from build123d import *

# Parameters (mm, degrees)
BOSS_EXTRUDE1_DEPTH = 20
FILLET1_R           = 50
FILLET2_R           = 5
SKETCH3_R           = 1.5
CUT_EXTRUDE1_DEPTH  = 20
SKETCH4_R           = 2.5
CUT_EXTRUDE2_DEPTH  = 10
SKETCH5_R           = 1
CUT_EXTRUDE3_DEPTH  = 20


with BuildPart() as part:
    # Sketch2 → Boss-Extrude1 (new body)
    with BuildSketch(Plane(origin=(0, 0, 0), x_dir=(1, 0, 0), z_dir=(0, 1, 0))):
        with BuildLine():
            Line((25, -30), (60, -30))
            Line((60, -30), (60, 0))
            Line((60, 0), (45, 0))
            Line((45, 0), (0, 10))
            Line((0, 10), (-45, 0))
            Line((-45, 0), (-60, 0))
            Line((-60, 0), (-60, -30))
            Line((-60, -30), (-25, -30))
            add(Edge.make_bspline(
                [(0, 0), (-26.0775505, -1.658562804), (-25, -30)],
                knots=[0, 0, 0, 1, 1, 1], degree=2))
            add(Edge.make_bspline(
                [(0, 0), (26.0775505, -1.658562804), (25, -30)],
                knots=[0, 0, 0, 1, 1, 1], degree=2))
        make_face()
    extrude(amount=BOSS_EXTRUDE1_DEPTH)

    # Fillet1
    fillet1_edges = [part.edges().sort_by_distance(p)[0] for p in [
        (0, 10, -10),
    ]]
    fillet(fillet1_edges, radius=FILLET1_R)

    # Fillet2
    fillet2_edges = [part.edges().sort_by_distance(p)[0] for p in [
        (-60, 10, 0),
        (60, 10, 0),
    ]]
    fillet(fillet2_edges, radius=FILLET2_R)

    # Sketch3 → Cut-Extrude1 (cut)
    with BuildSketch(Plane.XY.offset(30)):
        with Locations((50, 10)):
            Circle(SKETCH3_R)
    cut_extrude1 = extrude(amount=-CUT_EXTRUDE1_DEPTH, mode=Mode.SUBTRACT)

    # Sketch4 → Cut-Extrude2 (cut)
    with BuildSketch(Plane(origin=(0, 0, 0), x_dir=(-1, 0, 0), z_dir=(0, 0, -1))):
        with Locations((-50, 10)):
            Circle(SKETCH4_R)
    cut_extrude2 = extrude(amount=-CUT_EXTRUDE2_DEPTH, mode=Mode.SUBTRACT)

    # Mirror1: Cut-Extrude1, Cut-Extrude2 across plane
    add(cut_extrude1.mirror(Plane(origin=(0, 0, 0), x_dir=(0, 0, 1), z_dir=(1, 0, 0))), mode=Mode.SUBTRACT)
    add(cut_extrude2.mirror(Plane(origin=(0, 0, 0), x_dir=(0, 0, 1), z_dir=(1, 0, 0))), mode=Mode.SUBTRACT)

    # Sketch5 → Cut-Extrude3 (cut)
    with BuildSketch(Plane(origin=(0, 20, 0), x_dir=(1, 0, 0), z_dir=(0, 1, 0))):
        with Locations(Location((30, -27, 0), (0, 0, 270))):
            Circle(SKETCH5_R)
    cut_extrude3 = extrude(amount=-CUT_EXTRUDE3_DEPTH, mode=Mode.SUBTRACT)

    # Mirror2: Cut-Extrude3 across plane
    add(cut_extrude3.mirror(Plane(origin=(0, 0, 0), x_dir=(0, 0, 1), z_dir=(1, 0, 0))), mode=Mode.SUBTRACT)


solid = part.part
Build history of the part. All positions in model axes, mm. A direction names the side the tool comes from. Coordinates: 2 decimals unless noted, no trailing zeros. Write each loop counter-clockwise with the first axis right and the second up, starting at its lowest first coordinate (ties: lowest second). Pieces come first, ordered by that corner, then holes.
(1) 3-axis set-ups, long thin cutter, end or side, ignore diameter. For faces 5 (the cylindrical face through (-47.69, 9.04, 4.93)), 6 (the flat face through (60, 10, 18)): which of +Z, -Z, +X, -X, +Y, -Y reach the whole face in a straight line?
(2) Cut at A-A on x = -50. List the corners of the cut face in (y, z), and give its area (3 significant figures).
(3) Cut at B-B on y = 10. State how many separate pieces and enclosed holes the cut face has, and give its area (3 significant figures).
(4) Pin check, flat tips, straight feed: pin 1 Ø5 at (x, y) = (51.5, 7) entering from -Z; pin 2 Ø12 at (x, y) = (-5.5, 2.5) entering from -Z; pin 3 Ø12 at (y, z) = (10, -2.5) entering from -X; pin 4 Ø12 at (x, z) = (20, 21) entering from -Y. Stop position of each tip, or through.
(5) Mould opens along Y. For faces 1 (the cylindrical face through (47.69, 9.04, 4.93)), 2 (the flat face through (-48.8, 7.6, 0)), 3 (the flat face through (50, 8, 10)), 4 (the flat face through (-1, 20, -3)) say: pulls with the +Y half, pulls with the -Y half, needs draft (parallel to the pull), parting line crosses it, or undercut.
(6) Drill centre lines: line 1 (Y direction, x = 50, z = 4); line 2 (Y direction, x = -50, z = 20.25); line 3 (X direction, y = 11.25, z = 23). Where is each one in solid material? Low to high.
Working result:
1. face 5: -Z
1. face 6: +Z, -Z, +X, +Y, -Y
2. outline: (0, 0) - (7.5, 0) - (7.5, 10) - (8.5, 10) - (8.5, 30) - (0, 30) - close; (11.5, 10) - (12.5, 10) - (12.5, 0) - (20, 0) - (20, 30) - (11.5, 30) - close
2. area: 490 mm2
3. separate pieces: 3
3. enclosed holes: 2
3. area: 2,560 mm2
4. pin 1: stops at z = 0
4. pin 2: stops at z = -8.78
4. pin 3: stops at x = -59.77
4. pin 4: stops at y = 0
5. face 1: undercut
5. face 2: needs draft
5. face 3: undercut
5. face 4: pulls with the +Y half
6. line 1: y = 0 to 7.5, 12.5 to 20
6. line 2: y = 0 to 8.5, 11.5 to 20
6. line 3: x = -60 to -50.83, -49.17 to -24.81, 24.81 to 49.17, 50.83 to 60
